Answer from the drawing. Dimensions are ordinates in mm from the lowest x, y and z of the part. Coordinates: 2 decimals unless noted, no trailing zeros. Order: outer loops, then holes, each group sorted by start corner. A loop starts at its lowest first (then second) coordinate and runs counter-clockwise, first axis right, second up. Notation, with made-up numbers: (68, 61.5) -> (103, 61.5) arc R25 ccw to (103, 84.5) -> close; hole circle Ø5 at (64.5, 69.25). An arc over 180 degrees is marked (long way). Answer in a Markdown table with one row per item.
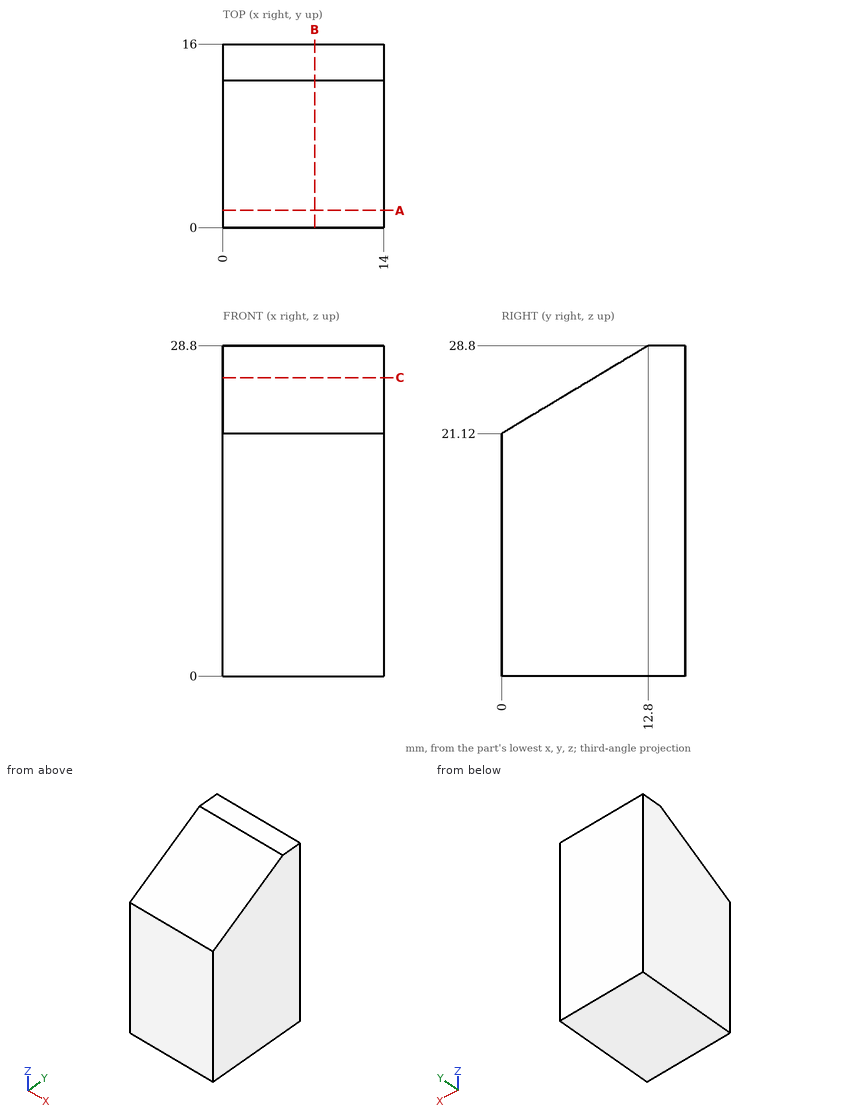
Q1. The part is cut by section B-B (x = 8). Write down the section's boundary in (y, z).
Outcome:
| item | result |
|---|---|
| outline | (0, 0) -> (16, 0) -> (16, 28.8) -> (12.8, 28.8) -> (0, 21.12) -> close |
Q2. Consider line 1 (Z direction, x = 9, y = 1); line 2 (Y direction, x = 2.5, z = 21.5); line 3 (Z direction, x = 6.25, y = 7.75). Determine where each line is inside the solid, lowest interval first.
Outcome:
| item | result |
|---|---|
| line 1 | 0 to 21.72 |
| line 2 | 0.63 to 16 |
| line 3 | 0 to 25.77 |
Q3. The part is cut by section C-C (z = 26). Write down the section's boundary in (x, y).
Outcome:
| item | result |
|---|---|
| outline | (0, 8.13) -> (14, 8.13) -> (14, 16) -> (0, 16) -> close |
Q4. The part is cut by section A-A (y = 1.5). Write down the section's boundary in (x, z).
Outcome:
| item | result |
|---|---|
| outline | (0, 0) -> (14, 0) -> (14, 22.02) -> (0, 22.02) -> close |
